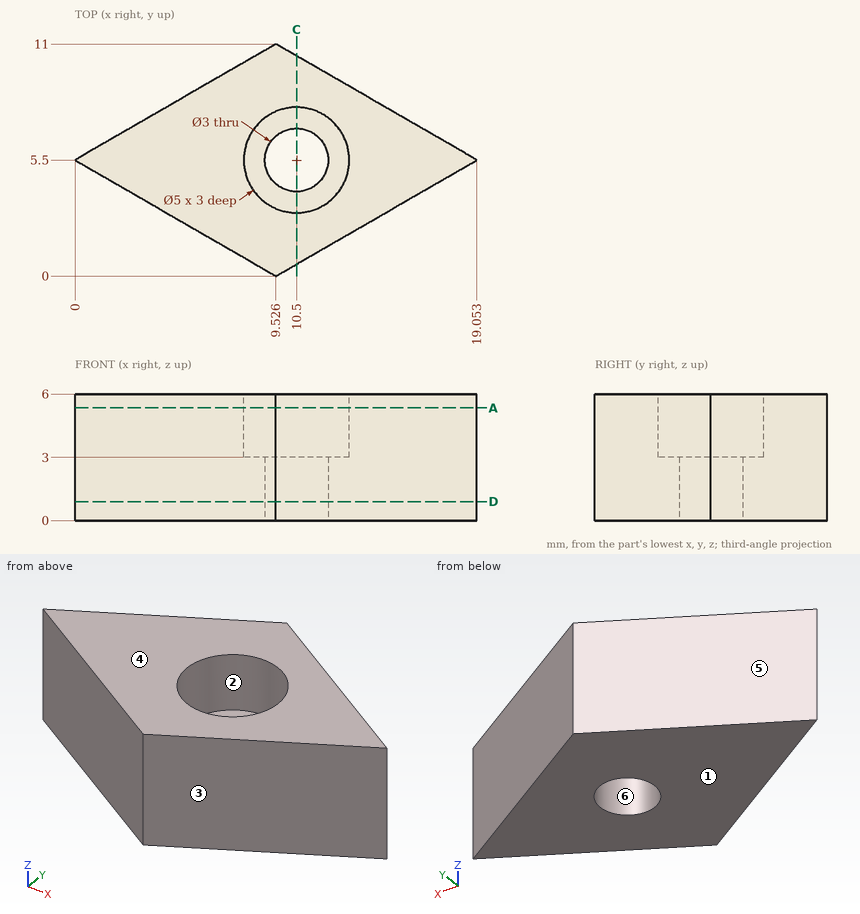
Job drawing, mm, ordinate dimensions from the low corner. One solid piece. A direction names the side the tool comes from. Give positions to 0.01 mm unless a question says otherwise; leave off trailing zeros. Loops run counter-clockwise (first coordinate to the right, second up) from the corner with the lowest first, then second, coordinate; pieces in that order, holes last.
Item 1: Pull direction X, two halves, no side cores. Call the marked faces 3, 4, 5 and 6: released by +X, released by -X, zero draft, split by the parting line, or undercut.
Answers follow:
face 3: released by +X
face 4: zero draft
face 5: released by -X
face 6: undercut
Item 2: Which spindle directions (+Z, -Z, +X, -X, +Y, -Y) get a long thin tool onto all of the face, cutting with end or side? Do the marked faces 1 and 2. Say none if no direction does.
Answers follow:
face 1: -Z, +X, -X, +Y, -Y
face 2: +Z
Item 3: Slice it at C-C, the plane x = 10.5. List the corners of the cut face in (y, z).
Answers follow:
outline: (0.56, 0) - (4, 0) - (4, 3) - (3, 3) - (3, 6) - (0.56, 6) - close; (7, 0) - (10.44, 0) - (10.44, 6) - (8, 6) - (8, 3) - (7, 3) - close
Item 4: Drill centre lines: line 1 (Y direction, x = 9.5, z = 4.7) (1 decimal); line 2 (Z direction, x = 9.5, y = 7.75); line 3 (Y direction, x = 11, z = 3.25). Where is each one in solid material? Low to high.
Answers follow:
line 1: y = 0 to 3.2, 7.8 to 11
line 2: z = 0 to 3
line 3: y = 0.85 to 3.05, 7.95 to 10.15
Item 5: Slice it at A-A, the plane z = 5.35. List the corners of the cut face in (x, y).
Answers follow:
outline: (0, 5.5) - (9.53, 0) - (19.05, 5.5) - (9.53, 11) - close; hole circle Ø5 at (10.5, 5.5)
Item 6: Flat gauge pins, fed straight in: pin 1 (1.5 mm diameter, centred on x = 11, y = 6, fed in from +Z); pin 2 (4 mm diameter, centred on x = 10.5, y = 5.5, fed in from -Z); pin 3 (2 mm diameter, centred on y = 2.5, z = 1, fed in from -X) (1 decimal); pin 4 (3.5 mm diameter, centred on x = 10.5, y = 5.5, fed in from +Z). Where does each tip first touch, or does it go through?
Answers follow:
pin 1: passes through
pin 2: stops at z = 0
pin 3: stops at x = 3.5
pin 4: stops at z = 3
Item 7: Slice it at D-D, the plane z = 0.9. List the corners of the cut face in (x, y).
Answers follow:
outline: (0, 5.5) - (9.53, 0) - (19.05, 5.5) - (9.53, 11) - close; hole circle Ø3 at (10.5, 5.5)
